from build123d import *

# Parameters (mm, degrees)
F1_DEPTH = 25.4
F2_R     = 45.643757
F3_DEPTH = 63.5
F4_SIZE  = 5.08


with BuildPart() as f1:
    # F0 (on Front) → F1 (new body)
    with BuildSketch(Plane.XZ):
        Polygon((-74.051848, -4.042859), (-43.009737, -60.416748), (20.419583, -71.295593), (68.472541, -28.487402), (64.964279, 35.772383), (12.53659, 73.094834), (-49.331407, 55.375384), align=None)
    extrude(amount=F1_DEPTH)

    # F2 (on face) → F3 (join)
    with BuildSketch(Plane.XZ.offset(25.4)):
        Circle(F2_R)
    extrude(amount=F3_DEPTH)

    # F4
    f4_edges = [f1.edges().sort_by_distance(p)[0] for p in [
        (-45.643757, -88.9, 0),
    ]]
    chamfer(f4_edges, length=F4_SIZE)


solid = f1.part
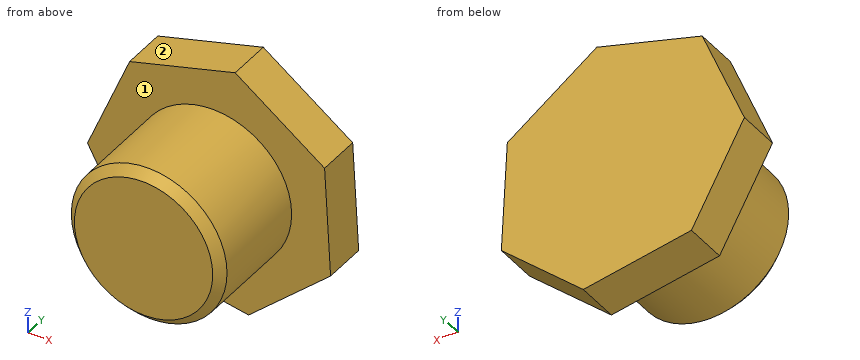
Verification items for the finished model (mm, model axes). Face numbers are marked on the shaded views. A direction names the side the tool comes from. Coordinates: 2 decimals unless noted, no trailing zeros. Order: outer loops, then holes, each group sorted by start corner. A loop starts at its lowest first (then second) coordinate and runs counter-clockwise, first axis right, second up. Notation, with made-up numbers: M 30,18 L 36,18 A26 ccw 36,43 Z; hole C 53.25,36 d6. An arc over 180 degrees is marked long. One line per item, written item: value. Start each with the question number.
Item 1: Sectioned sample at A-A on y = -13. Record the cut outline in (x, z), then the cut area to 3 significant figures.
Item 2: Sectioned sample at D-D on y = -75.5. Record the cut outline in (x, z).
Item 3: Thickness scan on probe 1 along Y at (x, z) = (29.5, -61); probe 2 along X at (y, z) = (-59.5, 21); probe 3 along Z at (x, y) = (-0.5, -84.5). Record the ranges inside material, lowest first.
Item 4: Sectioned sample at B-B on z = 0. Record the cut outline in (x, y).
Item 5: Depth check by flat-ended pin: P1, Ø5, axis at x = 42, y = -61, coming from the -Z side; P2, Ø4, axis at x = -16.5, y = -35.5, coming from the +Z side; P3, Ø1, axis at y = -25, z = -10.5, coming from the -X side. Enter the tip coordinate at first touch or a pass-through.
Item 6: Access from +Z, -Z, +X, -X, +Y, -Y to the whole of each face (thin tool, end or side, straight path). Record for the marked faces 1 and 2.
Item 7: Sectioned sample at C-C on x = 0. Record the cut outline in (y, z), then the cut area to 3 significant figures.
Calculated:
1. outline: M -74.05,-4.04 L -43.01,-60.42 L 20.42,-71.3 L 68.47,-28.49 L 64.96,35.77 L 12.54,73.09 L -49.33,55.38 Z
1. area: 15,100 mm^2
2. outline: C 0,0 d91.29
3. probe 1: -25.4 to 0
3. probe 2: -40.53 to 40.53
3. probe 3: -44.96 to 44.96
4. outline: M -72.37,-25.4 L -45.64,-25.4 L -45.64,-83.82 L -40.56,-88.9 L 40.56,-88.9 L 45.64,-83.82 L 45.64,-25.4 L 66.92,-25.4 L 66.92,0 L -72.37,0 Z
5. P1: z = -22.87
5. P2: z = 43.28
5. P3: x = -70.77
6. face 1: -Y
6. face 2: +Z, -X, +Y, -Y
7. outline: M -88.9,-40.56 L -83.82,-45.64 L -25.4,-45.64 L -25.4,-67.79 L 0,-67.79 L 0,69.5 L -25.4,69.5 L -25.4,45.64 L -83.82,45.64 L -88.9,40.56 Z
7. area: 9,260 mm^2
